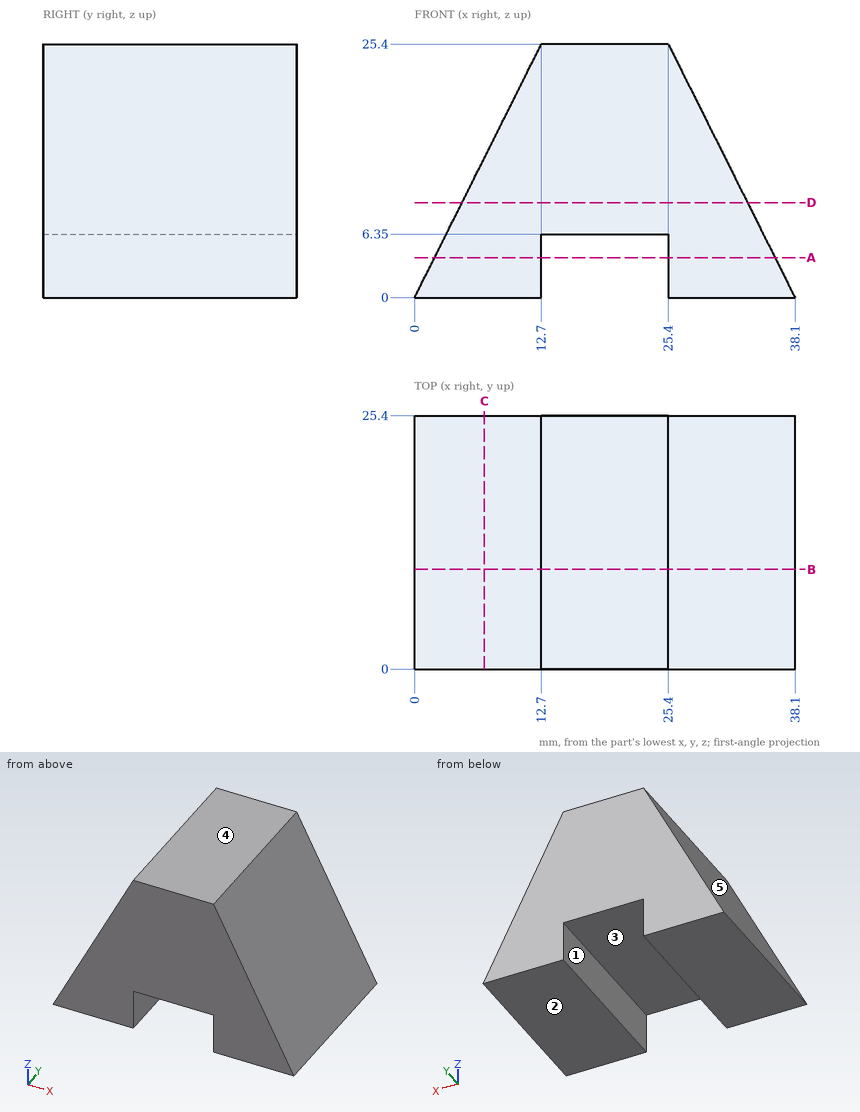
Check sheet for the drawn part. Datum: minimum x, y, z corner. Units: mm. A direction names the side the tool comes from. Round coordinates to 2 decimals unless told otherwise and drop trailing zeros. Write each loop counter-clockwise with the first axis right and the second up, starting at its lowest first coordinate (ties: lowest second). Pieces come first, ordered by that corner, then holes. Notation, with made-up numbers: (-29.5, 10) - (-2.5, 10) arc R24 ccw to (-2.5, 40) - close; hole circle Ø10 at (-7, -10). An arc over 180 degrees is marked (long way). Return JSON: item names as keys, results as strings.
Q1. Cross-section at A-A (z = 4). Record the boundary of the cut face in (x, y), then the cut area to 3 significant figures.
Returned:
{"outline": "(2, 0) - (12.7, 0) - (12.7, 25.4) - (2, 25.4) - close; (25.4, 0) - (36.1, 0) - (36.1, 25.4) - (25.4, 25.4) - close", "area": "544 mm²"}
Q2. Cross-section at D-D (z = 9.5). Record the boundary of the cut face in (x, y), then the cut area to 3 significant figures.
Returned:
{"outline": "(4.75, 0) - (33.35, 0) - (33.35, 25.4) - (4.75, 25.4) - close", "area": "726 mm²"}
Q3. Depth check by flat-ended pin: P1, Ø3, axis at y = 15, z = 2.5, coming from the +X side; P2, Ø6.5, axis at x = 19, y = 16, coming from the -Z side; P3, Ø7, axis at y = 16, z = 4, coming from the -X side. Enter the tip coordinate at first touch or a pass-through.
Returned:
{"P1": "stops at x = 37.6", "P2": "stops at z = 6.35", "P3": "stops at x = 0.25"}
Q4. Cross-section at C-C (x = 7). Record the boundary of the cut face in (y, z).
Returned:
{"outline": "(0, 0) - (25.4, 0) - (25.4, 14) - (0, 14) - close"}
Q5. Draft check along X on the marked faces 3, 4 and 5. Enter one of: released by +X, released by -X, zero draft, split by the parting line, or undercut.
Returned:
{"face 3": "undercut", "face 4": "zero draft", "face 5": "released by -X"}
Q6. Scan lines: L1, parallel to X at y = 8.5, z = 5.5; L2, parallel to Z at x = 23.5, y = 24.25; L3, parallel to X at y = 20.25, z = 6. Record each from-to range of solid material in increasing order. Write a range as from..to.
Returned:
{"L1": "x = 2.75..12.7, 25.4..35.35", "L2": "z = 6.35..25.4", "L3": "x = 3..12.7, 25.4..35.1"}
Q7. Access from +Z, -Z, +X, -X, +Y, -Y to the whole of each face (thin tool, end or side, straight path). Record for the marked faces 1 and 2.
Returned:
{"face 1": "-Z, +Y, -Y", "face 2": "-Z, +X, -X, +Y, -Y"}
Q8. Cross-section at B-B (y = 10). Record the boundary of the cut face in (x, z).
Returned:
{"outline": "(0, 0) - (12.7, 0) - (12.7, 6.35) - (25.4, 6.35) - (25.4, 0) - (38.1, 0) - (25.4, 25.4) - (12.7, 25.4) - close"}
